Here's the drawing with two shaded views (mm, measured from the low corner). I have some questions. A direction names the side the tool comes from. Round coordinates to 2 decimals unless told otherwise and drop trailing zeros. Loops run counter-clockwise (first coordinate to the right, second up) from the corner with the lowest first, then second, coordinate; pieces in that order, holes last.
(1) If I drill on line 1 along X through (y, z) = (5.5, 10.5) (1 decimal); line 2 along X through (y, z) = (13.75, 13) (1 decimal); line 3 along Y through (x, z) = (25, 32), over which ranges is the centre line in solid material (lowest first)?
(2) I want a section at A-A on x = 85.5. Write out the boundary of the cut face in (y, z) (1 decimal), plus the area to 3 significant figures.
(3) Which directions (+Z, -Z, +X, -X, +Y, -Y) give clear straight access to the entire face, cutting with the end or side of a thin tool? Please do the marked faces 1, 2 and 3.
(4) I want a section at D-D on z = 30. Write out the boundary of the cut face in (x, y) (1 decimal), plus the area to 3 significant figures.
(5) Will these pins go through, and if not, where does the flat tip stop? pin 1 Ø14 at (x, z) = (44, 29.5) entering from +Y; pin 2 Ø3 at (x, z) = (5.4, 11.28) entering from -Y; pin 3 Ø4.5 at (x, z) = (84.77, 11.28) entering from +Y; pin 4 Ø3 at (x, y) = (69, 4.5) entering from +Z.
(6) Thinking about a two-plate mould opening in X: for the marked faces 4, 5, 6 and 7, which applies, released by +X, released by -X, zero draft, split by the parting line, or undercut?
(7) I want a section at B-B on y = 16. Write out the boundary of the cut face in (x, z).
(8) I want a section at C-C on x = 66. Write out the boundary of the cut face in (y, z), plus the area to 3 significant figures.
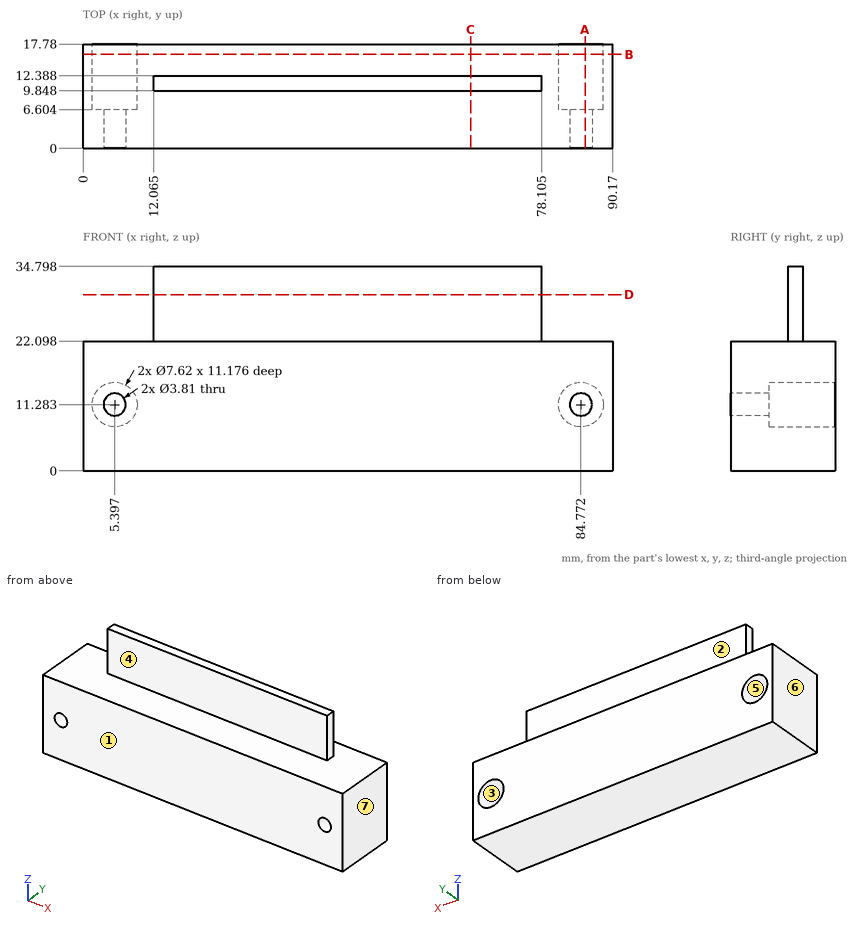
Filled sheet:
1. line 1: x = 0 to 3.7, 7.1 to 83, 86.5 to 90.2
1. line 2: x = 0 to 2, 8.8 to 81.4, 88.2 to 90.2
1. line 3: y = 9.85 to 12.39
2. outline: (0, 0) - (17.8, 0) - (17.8, 7.5) - (6.6, 7.5) - (6.6, 9.5) - (0, 9.5) - close; (0, 13) - (6.6, 13) - (6.6, 15) - (17.8, 15) - (17.8, 22.1) - (0, 22.1) - close
2. area: 286 mm2
3. face 1: +Z, -Z, +X, -X, -Y
3. face 2: +Z, +X, -X, +Y
3. face 3: +Y
4. outline: (12.1, 9.8) - (78.1, 9.8) - (78.1, 12.4) - (12.1, 12.4) - close
4. area: 168 mm2
5. pin 1: stops at y = 12.39
5. pin 2: passes through
5. pin 3: stops at y = 6.6
5. pin 4: stops at z = 22.1
6. face 4: zero draft
6. face 5: undercut
6. face 6: released by -X
6. face 7: released by +X
7. outline: (0, 0) - (90.17, 0) - (90.17, 22.1) - (0, 22.1) - close; hole circle Ø7.62 at (5.4, 11.28); hole circle Ø7.62 at (84.77, 11.28)
8. outline: (0, 0) - (17.78, 0) - (17.78, 22.1) - (12.39, 22.1) - (12.39, 34.8) - (9.85, 34.8) - (9.85, 22.1) - (0, 22.1) - close
8. area: 425 mm2
